Can you work these out from the model? Positions are in its coordinate system, mm. Face numbers are marked on the shaded views. A direction names the side the tool comes from. Give positions to 0.01 mm unless a question says otherwise; leave off trailing zeros. Write each loop counter-clockwise with the first axis right and the second up, starting at its lowest first coordinate (ties: lowest second). Pieces come first, ordered by that corner, then holes.
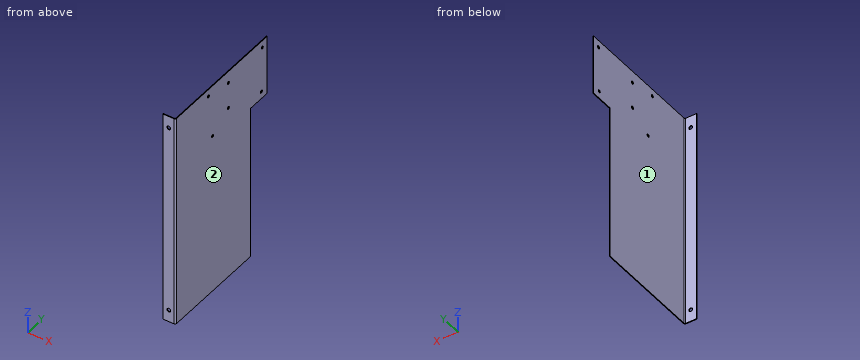
```python
from build123d import *

# Parameters (mm, degrees)
BASE_FLANGE1_DEPTH = 228.6
CUT_EXTRUDE1_REACH = 270.245
SKETCH4_W          = 165.1
SKETCH4_H          = 25.4
CUT_EXTRUDE2_REACH = 270.245
SKETCH6_R          = 2
SKETCH7_R          = 1.5621
CUT_EXTRUDE3_DEPTH = 269.244677605


# Sheet-metal steps are written as plain solids
with BuildPart() as part:
    # Sketch1 → Base-Flange1 (new body)
    with BuildSketch(Plane.XY):
        with BuildLine():
            Line((0, 0), (11.7, 0))
            ThreePointArc((11.7, 0), (12.407106781, 0.292893219), (12.7, 1))
            Line((12.7, 1), (12.7, 139.7))
            Line((12.7, 139.7), (13.45946, 139.7))
            Line((13.45946, 139.7), (13.45946, 1))
            ThreePointArc((13.45946, 1), (12.944126097, -0.244126097), (11.7, -0.75946))
            Line((11.7, -0.75946), (0, -0.75946))
            Line((0, -0.75946), (0, 0))
        make_face()
    extrude(amount=BASE_FLANGE1_DEPTH)

    # Sketch4 → Cut-Extrude1 (cut, up to next)
    with BuildSketch(Plane(origin=(13.45946, 0, 0), x_dir=(0, 0, -1), z_dir=(1, 0, 0)), mode=Mode.PRIVATE) as cut_extrude1_sk1:
        with Locations((-82.55, 127)):
            Rectangle(SKETCH4_W, SKETCH4_H)
    cut_extrude1_tool1 = extrude(cut_extrude1_sk1.sketch, amount=-CUT_EXTRUDE1_REACH, mode=Mode.PRIVATE) & part.part
    add(cut_extrude1_tool1.solids().sort_by_distance((13.45946, 127, 82.55))[0], mode=Mode.SUBTRACT)

    # Sketch6 → Cut-Extrude2 (cut, up to next)
    with BuildSketch(Plane(origin=(0, 0, 0), x_dir=(1, 0, 0), z_dir=(0, 1, 0)), mode=Mode.PRIVATE) as cut_extrude2_sk1:
        with Locations(Location((6.35, -12.7, 0), (0, 0, 270))):
            Circle(SKETCH6_R)
    cut_extrude2_tool1 = extrude(cut_extrude2_sk1.sketch, amount=-CUT_EXTRUDE2_REACH, mode=Mode.PRIVATE) & part.part
    # Sketch6 → Cut-Extrude2 (cut, up to next)
    with BuildSketch(Plane(origin=(0, 0, 0), x_dir=(1, 0, 0), z_dir=(0, 1, 0)), mode=Mode.PRIVATE) as cut_extrude2_sk2:
        with Locations(Location((6.35, -215.9, 0), (0, 0, 270))):
            Circle(SKETCH6_R)
    cut_extrude2_tool2 = extrude(cut_extrude2_sk2.sketch, amount=-CUT_EXTRUDE2_REACH, mode=Mode.PRIVATE) & part.part
    add(cut_extrude2_tool1.solids().sort_by_distance((6.35, 0, 12.7))[0], mode=Mode.SUBTRACT)
    add(cut_extrude2_tool2.solids().sort_by_distance((6.35, 0, 215.9))[0], mode=Mode.SUBTRACT)

    # Sketch7 → Cut-Extrude3 (cut, through all)
    with BuildSketch(Plane(origin=(13.45946, 0, 0), x_dir=(0, 0, -1), z_dir=(1, 0, 0))):
        with Locations((-221.0181, 49.61814)):
            Circle(SKETCH7_R)
        with Locations((-172.7581, 55.96814)):
            Circle(SKETCH7_R)
        with Locations((-215.9381, 80.09814)):
            Circle(SKETCH7_R)
        with Locations((-187.9981, 80.09814)):
            Circle(SKETCH7_R)
        with Locations((-221.0181, 132.16814)):
            Circle(SKETCH7_R)
        with Locations((-172.7581, 130.89814)):
            Circle(SKETCH7_R)
    extrude(amount=-CUT_EXTRUDE3_DEPTH, mode=Mode.SUBTRACT)


solid = part.part
```
1) Suppose I cut it at A-A on z = 158. Write out the boundary of the cut face in (x, y).
Values follow:
outline: (0, -0.76) - (11.7, -0.76) arc R1.76 ccw to (13.46, 1) - (13.46, 114.3) - (12.7, 114.3) - (12.7, 1) arc R1 cw to (11.7, 0) - (0, 0) - close
2) For pin 1 Ø4 at (y, z) = (130.9, 172.76) entering from -X; pin 2 Ø8 at (x, z) = (5, 74.5) entering from +Y; pin 3 Ø0.8 at (x, z) = (13, 51) entering from +Y, each with a flat end and sliding along its axis, tell me the tip position at first contact or that it passes through.
Values follow:
pin 1: stops at x = 12.7
pin 2: stops at y = 0
pin 3: stops at y = 114.3
3) Suppose I cut it at B-B on y = 90. Write out the boundary of the cut face in (x, z), plus the area to 3 significant figures.
Values follow:
outline: (12.7, 0) - (13.46, 0) - (13.46, 228.6) - (12.7, 228.6) - close
area: 174 mm2
4) Please list where these lines run through material, in increasing order: L1, parallel to X at y = 115.5, z = 167.5; L2, parallel to Y at x = 3.5, z = 177; L3, parallel to Z at x = 13.25, y = 133.
Values follow:
L1: x = 12.7 to 13.46
L2: y = -0.76 to 0
L3: z = 165.1 to 219.7, 222.34 to 228.6
5) Suppose I cut it at C-C on z = 205. Write out the boundary of the cut face in (x, y).
Values follow:
outline: (0, -0.76) - (11.7, -0.76) arc R1.76 ccw to (13.46, 1) - (13.46, 139.7) - (12.7, 139.7) - (12.7, 1) arc R1 cw to (11.7, 0) - (0, 0) - close
6) For the marked faces 1 and 2, which set-ups out of +Z, -Z, +X, -X, +Y, -Y let a thin tool reach every point of the face, with its end or its side?
Values follow:
face 1: +Z, -Z, -X, +Y
face 2: +Z, -Z, +X, +Y, -Y
